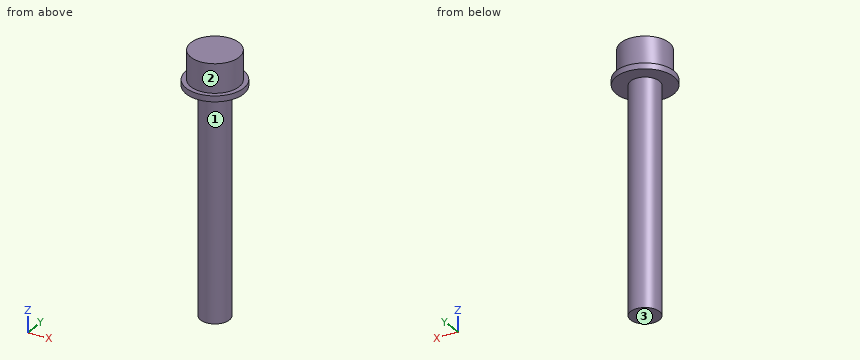
```python
from build123d import *

# Parameters (mm, degrees)
F0_R     = 2.5
F1_DEPTH = 40
F2_R     = 4.2
F3_DEPTH = 5
F4_R     = 5
F5_DEPTH = 1


with BuildPart() as f1:
    # F0 (on Top) → F1 (new body)
    with BuildSketch(Plane.XY):
        Circle(F0_R)
    extrude(amount=-F1_DEPTH)

    # F2 (on Top) → F3 (join)
    with BuildSketch(Plane.XY):
        Circle(F2_R)
    extrude(amount=F3_DEPTH)

    # F4 (on Top) → F5 (join)
    with BuildSketch(Plane.XY):
        Circle(F4_R)
    extrude(amount=-F5_DEPTH)


solid = f1.part
```
Verification items for the finished model (mm, model axes). Face numbers are marked on the shaded views. A direction names the side the tool comes from. Coordinates: 2 decimals unless noted, no trailing zeros. Loops run counter-clockwise (first coordinate to the right, second up) from the corner with the lowest first, then second, coordinate; pieces in that order, holes last. Notation, with made-up numbers: (47, -1.75) - (66, -1.75) arc R18 ccw to (66, 30.25) - close; hole circle Ø1 at (-37, 81.5). An arc over 180 degrees is marked (long way). Put each result on its own line as item: value.
Item 1: Scan lines: line 1 along Z through (x, y) = (-2.5, -2); line 2 along Z through (x, y) = (-1.75, 4); line 3 along Y through (x, z) = (1, -5.5). Record each from-to range of solid material in increasing order.
Conclusion:
line 1: z = -1 to 5
line 2: z = -1 to 0
line 3: y = -2.29 to 2.29
Item 2: Section check C-C (z = -10). Enter the section's corners in (x, y).
Conclusion:
outline: circle Ø5 at (0, 0)
Item 3: Set-up check for the marked faces 1, 2 and 3: record each of +Z, -Z, +X, -X, +Y, -Y from which the full face is reachable in a straight line by a thin tool's end or side.
Conclusion:
face 1: -Z
face 2: +Z
face 3: -Z, +X, -X, +Y, -Y
Item 4: Section check A-A (y = 0). Enter the section's corners in (x, z), then the cut area to 3 significant figures.
Conclusion:
outline: (-5, -1) - (-2.5, -1) - (-2.5, -40) - (2.5, -40) - (2.5, -1) - (5, -1) - (5, 0) - (4.2, 0) - (4.2, 5) - (-4.2, 5) - (-4.2, 0) - (-5, 0) - close
area: 247 mm2
Item 5: Section check D-D (x = 3.25). Enter the section's corners in (y, z).
Conclusion:
outline: (-3.8, -1) - (3.8, -1) - (3.8, 0) - (2.66, 0) - (2.66, 5) - (-2.66, 5) - (-2.66, 0) - (-3.8, 0) - close
Item 6: Gauge pin test, flat ends, axial feed: pin 1 Ø1 at (x, y) = (3.5, -4) entering from -Z; pin 2 Ø4 at (x, z) = (-0.5, -10.5) entering from +Y; pin 3 Ø2 at (x, z) = (1, -19.5) entering from -Y. Record the tip position at first contact, or that the pin passes through.
Conclusion:
pin 1: stops at z = -1
pin 2: stops at y = 2.5
pin 3: stops at y = -2.5
